from build123d import *

# Parameters (mm, degrees)
SKETCH2_R           = 32.2072
BOSS_EXTRUDE1_DEPTH = 109.601
CHAMFER1_SIZE       = 1.27
CHAMFER2_SIZE       = 1.27
SKETCH3_R           = 9.525
BOSS_EXTRUDE2_DEPTH = 3.9878
SKETCH4_R           = 3.96875
BOSS_EXTRUDE3_DEPTH = 31.623
CHAMFER3_SIZE       = 1.27
CHAMFER4_SIZE       = 1.27
SKETCH5_R           = 15.24
BOSS_EXTRUDE4_DEPTH = 3.9878
CHAMFER5_SIZE       = 1.27
CUT_EXTRUDE1_DEPTH  = 1.15062
SKETCH7_R           = 2.413
CUT_EXTRUDE2_DEPTH  = 6.35


with BuildPart() as part:
    # Sketch2 → Boss-Extrude1 (new body)
    with BuildSketch(Plane(origin=(0, 0, 0), x_dir=(0, 0, -1), z_dir=(1, 0, 0))):
        Circle(SKETCH2_R)
    extrude(amount=BOSS_EXTRUDE1_DEPTH)

    # Chamfer1
    chamfer1_edges = [part.edges().sort_by_distance(p)[0] for p in [
        (0, 0, 32.2072),
    ]]
    chamfer(chamfer1_edges, length=CHAMFER1_SIZE)

    # Chamfer2
    chamfer2_edges = [part.edges().sort_by_distance(p)[0] for p in [
        (109.601, 0, 32.2072),
    ]]
    chamfer(chamfer2_edges, length=CHAMFER2_SIZE)

    # Sketch3 → Boss-Extrude2 (add)
    with BuildSketch(Plane(origin=(109.601, 0, 0), x_dir=(0, 0, -1), z_dir=(1, 0, 0))):
        Circle(SKETCH3_R)
    extrude(amount=BOSS_EXTRUDE2_DEPTH)

    # Sketch4 → Boss-Extrude3 (add)
    with BuildSketch(Plane(origin=(113.5888, 0, 0), x_dir=(0, 0, -1), z_dir=(1, 0, 0))):
        Circle(SKETCH4_R)
    extrude(amount=BOSS_EXTRUDE3_DEPTH)

    # Chamfer3
    chamfer3_edges = [part.edges().sort_by_distance(p)[0] for p in [
        (113.5888, 0, 9.525),
    ]]
    chamfer(chamfer3_edges, length=CHAMFER3_SIZE)

    # Chamfer4
    chamfer4_edges = [part.edges().sort_by_distance(p)[0] for p in [
        (145.2118, 0, 3.96875),
    ]]
    chamfer(chamfer4_edges, length=CHAMFER4_SIZE)

    # Sketch5 → Boss-Extrude4 (add)
    with BuildSketch(Plane.ZY):
        Circle(SKETCH5_R)
    extrude(amount=BOSS_EXTRUDE4_DEPTH)

    # Chamfer5
    chamfer5_edges = [part.edges().sort_by_distance(p)[0] for p in [
        (-3.9878, 0, -15.24),
    ]]
    chamfer(chamfer5_edges, length=CHAMFER5_SIZE)

    # Sketch6 → Cut-Extrude1 (cut)
    with BuildSketch(Plane.XY.offset(3.96875)):
        with BuildLine():
            Line((120.58269, 0.99949), (138.68273, 0.99949))
            ThreePointArc((138.68273, 0.99949), (139.68222, 0), (138.68273, -0.99949))
            Line((138.68273, -0.99949), (120.58269, -0.99949))
            ThreePointArc((120.58269, -0.99949), (119.5832, 0), (120.58269, 0.99949))
        make_face()
    extrude(amount=-CUT_EXTRUDE1_DEPTH, mode=Mode.SUBTRACT)

    # Sketch7 → Cut-Extrude2 (cut)
    with BuildSketch(Plane(origin=(109.601, 0, 0), x_dir=(0, 0, -1), z_dir=(1, 0, 0))):
        with Locations((0, 25.4)):
            Circle(SKETCH7_R)
        with Locations((25.4, 0)):
            Circle(SKETCH7_R)
        with Locations((0, -25.4)):
            Circle(SKETCH7_R)
        with Locations((-25.4, 0)):
            Circle(SKETCH7_R)
    extrude(amount=-CUT_EXTRUDE2_DEPTH, mode=Mode.SUBTRACT)


solid = part.part
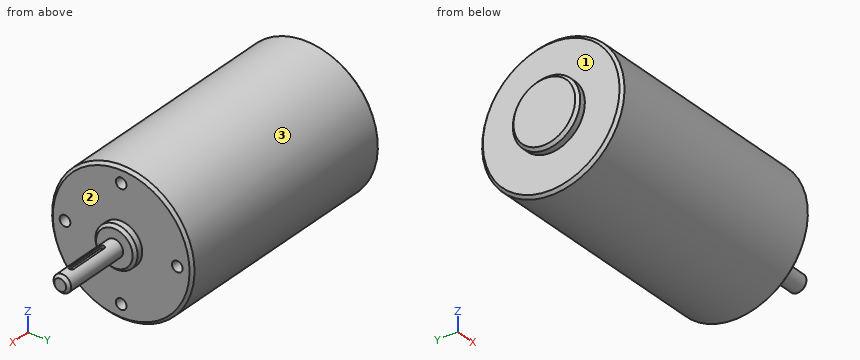
CAD build for the part. Positions are in the model's coordinates, mm. Face numbers are marked on the shaded views. A direction names the side the tool comes from. Coordinates: 2 decimals unless noted, no trailing zeros. Write each loop counter-clockwise with the first axis right and the second up, starting at its lowest first coordinate (ties: lowest second). Pieces come first, ordered by that corner, then holes. Notation, with made-up numbers: M 46,38 L 95,38 A32 ccw 95,70 Z; hole C 1.5,8 d1. An arc over 180 degrees is marked long. Answer as a JSON object with one key per item and string values. Group by question number.
1) Tool access for the marked faces 1, 2 and 3: list every direction of +Z, -Z, +X, -X, +Y, -Y with a clear straight run to the whole face (end or side of a thin tool).
2) Wall check: line 1 (Y direction, x = 107.25, z = 0); line 2 (X direction, y = -12.5, z = -17); line 3 (Y direction, x = 104.75, z = -25.4). Give the ranges that are in metal, low to high. Write a range as from..to.
3) Pin check, flat tips, straight feed: pin 1 Ø4.5 at (y, z) = (-25.4, 0) entering from +X; pin 2 Ø8 at (x, z) = (70, -4) entering from +Y; pin 3 Ø5 at (x, z) = (61, -17.5) entering from +Y. Stop position of each tip, or through.
4) Saw through at B-B (x = 34.5). Write the cut outline in (y, z), plus the area to 3 significant figures.
Values follow:
{
 "1": {"face 1": "-X", "face 2": "+X", "face 3": "+X, -X"},
 "2": {"line 1": "y = -32.21..-27.81, -22.99..22.99, 27.81..32.21", "line 2": "x = 0..109.6", "line 3": "y = -19.8..-2.41, 2.41..19.8"},
 "3": {"pin 1": "stops at x = 103.25", "pin 2": "stops at y = 32.21", "pin 3": "stops at y = 28.5"},
 "4": {"outline": "C 0,0 d64.41", "area": "3,260 mm2"}
}
